from build123d import *

# Parameters (mm, degrees)
SKETCH1_W                = 2400
SKETCH1_H                = 225
BOSS_EXTRUDE1_DEPTH      = 10
BOSS_EXTRUDE2_START      = 30
BOSS_EXTRUDE2_DEPTH      = 80
BOSS_EXTRUDE3_START      = -30
BOSS_EXTRUDE3_DEPTH      = 80
BOSS_EXTRUDE4_DEPTH      = 110
BOSS_EXTRUDE4_DEPTH_BACK = 110
BOSS_EXTRUDE5_START      = -30
BOSS_EXTRUDE5_DEPTH      = 80


with BuildPart() as part:
    # Sketch1 → Boss-Extrude1 (new body)
    with BuildSketch(Plane(origin=(0, 0, 0), x_dir=(1, 0, 0), z_dir=(0, 1, 0))):
        Rectangle(SKETCH1_W, SKETCH1_H)
    extrude(amount=BOSS_EXTRUDE1_DEPTH)

    # Sketch2 → Boss-Extrude2 (add)
    with BuildSketch(Plane.XY.offset(BOSS_EXTRUDE2_START)):
        Polygon((425, 10), (450, 40), (575, 40), (600, 10), align=None)
    extrude(amount=BOSS_EXTRUDE2_DEPTH)

    # Sketch3 → Boss-Extrude3 (add)
    with BuildSketch(Plane.XY.offset(BOSS_EXTRUDE3_START)):
        Polygon((-50, 40), (-75, 10), (100, 10), (75, 40), align=None)
    extrude(amount=-BOSS_EXTRUDE3_DEPTH)

    # Sketch4 → Boss-Extrude4 (add, two sides: drawn at the far end of the back side and taken through both)
    with BuildSketch(Plane.XY.offset(-BOSS_EXTRUDE4_DEPTH_BACK)):
        Polygon((-550, 40), (-575, 10), (-400, 10), (-425, 40), align=None)
    extrude(amount=BOSS_EXTRUDE4_DEPTH + BOSS_EXTRUDE4_DEPTH_BACK)

    # Sketch5 → Boss-Extrude5 (add)
    with BuildSketch(Plane.XY.offset(BOSS_EXTRUDE5_START)):
        Polygon((-1050, 40), (-1075, 10), (-900, 10), (-925, 40), align=None)
    extrude(amount=-BOSS_EXTRUDE5_DEPTH)


solid = part.part
CAD build for the part. Positions are in the model's coordinates, mm. Give positions to 0.01 mm unless a question says otherwise; leave off trailing zeros. Write each loop counter-clockwise with the first axis right and the second up, starting at its lowest first coordinate (ties: lowest second). Pieces come first, ordered by that corner, then holes. Notation, with made-up numbers: M 53,30 L 83,30 A16 cw 83,48 Z; hole C -22,-34.75 d6. An arc over 180 degrees is marked long. Put each result on its own line as item: value. Start each with the question number.
(1) Flat gauge pins, fed straight in: pin 1 Ø4 at (y, z) = (27, 60) entering from +X; pin 2 Ø2 at (y, z) = (28, -54) entering from -X; pin 3 Ø4 at (y, z) = (22, 42) entering from -X. Where does each tip first touch, or does it go through?
(2) Probe L1, parallel to X at y = 38.5, z = -95; L2, parallel to X at y = 35, z = -48.5; L3, parallel to Y at x = 911, z = 37. List the from-to ranges inside material, lowest first.
(3) Band-saw the part on A-A, the plane y = 18. Write the cut outline in (x, z), and give its area (3 significant figures).
(4) Band-saw the part on C-C, the plane x = -467. Write the cut outline in (y, z).
(5) Band-saw the part on B-B, the plane z = 90. Write the cut outline in (x, y).
(6) Mould opens along X. For faces 1 (the face through (-17, 10, -2)), 2 (the face through (13, 40, -69)) say: +X half, -X half, draft (parallel to the pull), parting line (faces both ways), or undercut.
(7) Band-saw the part on D-D, the plane x = -1019. Write the cut outline in (y, z).
Response values:
1. pin 1: stops at x = 587.5
1. pin 2: stops at x = -1060.83
1. pin 3: stops at x = -566.67
2. L1: x = -1051.25 to -923.75, -551.25 to -423.75, -51.25 to 76.25
2. L2: x = -1054.17 to -920.83, -554.17 to -420.83, -54.17 to 79.17
2. L3: y = 0 to 10
3. outline: M -1068.33,-110 L -906.67,-110 L -906.67,-30 L -1068.33,-30 Z; M -568.33,-110 L -406.67,-110 L -406.67,110 L -568.33,110 Z; M -68.33,-110 L 93.33,-110 L 93.33,-30 L -68.33,-30 Z; M 431.67,30 L 593.33,30 L 593.33,110 L 431.67,110 Z
3. area: 74,400 mm2
4. outline: M 0,-112.5 L 10,-112.5 L 10,-110 L 40,-110 L 40,110 L 10,110 L 10,112.5 L 0,112.5 Z
5. outline: M -1200,0 L 1200,0 L 1200,10 L 600,10 L 575,40 L 450,40 L 425,10 L -400,10 L -425,40 L -550,40 L -575,10 L -1200,10 Z
6. face 1: undercut
6. face 2: draft
7. outline: M 0,-112.5 L 10,-112.5 L 10,-110 L 40,-110 L 40,-30 L 10,-30 L 10,112.5 L 0,112.5 Z
